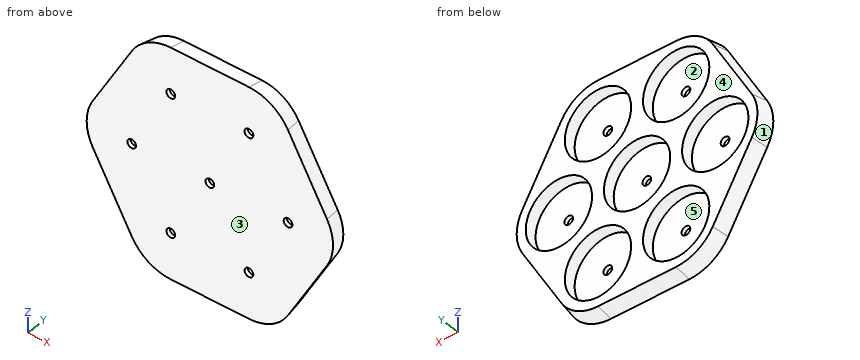
from build123d import *

# Parameters (mm, degrees)
BOSS_EXTRUDE1_DEPTH = 4
BOSS_EXTRUDE1_TAPER = 10
CUT_EXTRUDE1_START  = 4
SKETCH1_3_R         = 1.1
CUT_EXTRUDE1_DEPTH  = 4
CUT_EXTRUDE2_START  = 4
SKETCH1_4_R         = 8.4
SKETCH1_4_R_2       = 1.1
CUT_EXTRUDE2_DEPTH  = 3


with BuildPart() as part:
    # Sketch1 → Boss-Extrude1 (new body)
    with BuildSketch(Plane(origin=(0, 0, 0), x_dir=(1, 0, 0), z_dir=(0, 1, 0))):
        with BuildLine():
            ThreePointArc((-29.7, 28.547302995), (-35.4, 27.019992598), (-39.572689603, 22.847302995))
            Line((-39.572689603, 22.847302995), (-49.472689603, 5.7))
            ThreePointArc((-49.472689603, 5.7), (-51, 0), (-49.472689603, -5.7))
            Line((-49.472689603, -5.7), (-39.572689603, -22.847302995))
            ThreePointArc((-39.572689603, -22.847302995), (-35.4, -27.019992598), (-29.7, -28.547302995))
            Line((-29.7, -28.547302995), (-9.9, -28.547302995))
            ThreePointArc((-9.9, -28.547302995), (-4.2, -27.019992598), (-0.027310397, -22.847302995))
            Line((-0.027310397, -22.847302995), (9.872689603, -5.7))
            ThreePointArc((9.872689603, -5.7), (11.4, 0), (9.872689603, 5.7))
            Line((9.872689603, 5.7), (-0.027310397, 22.847302995))
            ThreePointArc((-0.027310397, 22.847302995), (-4.2, 27.019992598), (-9.9, 28.547302995))
            Line((-9.9, 28.547302995), (-29.7, 28.547302995))
        make_face()
    extrude(amount=BOSS_EXTRUDE1_DEPTH, taper=BOSS_EXTRUDE1_TAPER)

    # Sketch1<3> → Cut-Extrude1 (cut)
    with BuildSketch(Plane(origin=(0, 0, 0), x_dir=(1, 0, 0), z_dir=(0, 1, 0)).offset(CUT_EXTRUDE1_START)):
        with Locations(Location((-9.9, -17.147302995, 0), (0, 0, 270))):
            Circle(SKETCH1_3_R)
        with Locations(Location((0, 0, 0), (0, 0, 270))):
            Circle(SKETCH1_3_R)
        with Locations(Location((-29.7, -17.147302995, 0), (0, 0, 270))):
            Circle(SKETCH1_3_R)
        with Locations(Location((-39.6, 0, 0), (0, 0, 270))):
            Circle(SKETCH1_3_R)
        with Locations(Location((-9.9, 17.147302995, 0), (0, 0, 270))):
            Circle(SKETCH1_3_R)
        with Locations(Location((-29.7, 17.147302995, 0), (0, 0, 270))):
            Circle(SKETCH1_3_R)
        with Locations(Location((-19.8, 0, 0), (0, 0, 270))):
            Circle(SKETCH1_3_R)
    extrude(amount=-CUT_EXTRUDE1_DEPTH, mode=Mode.SUBTRACT)

    # Sketch1<4> → Cut-Extrude2 (cut)
    # profile 1 of 7: a face of its own
    with BuildSketch(Plane(origin=(0, 0, 0), x_dir=(1, 0, 0), z_dir=(0, 1, 0)).offset(CUT_EXTRUDE2_START)):
        with Locations(Location((-19.8, 0, 0), (0, 0, 270))):
            Circle(SKETCH1_4_R)
        with Locations(Location((-19.8, 0, 0), (0, 0, 270))):
            Circle(SKETCH1_4_R_2, mode=Mode.SUBTRACT)
    # profile 2 of 7: a face of its own
    with BuildSketch(Plane(origin=(0, 0, 0), x_dir=(1, 0, 0), z_dir=(0, 1, 0)).offset(CUT_EXTRUDE2_START)):
        with Locations(Location((-9.9, -17.147302995, 0), (0, 0, 270))):
            Circle(SKETCH1_4_R)
        with Locations(Location((-9.9, -17.147302995, 0), (0, 0, 270))):
            Circle(SKETCH1_4_R_2, mode=Mode.SUBTRACT)
    # profile 3 of 7: a face of its own
    with BuildSketch(Plane(origin=(0, 0, 0), x_dir=(1, 0, 0), z_dir=(0, 1, 0)).offset(CUT_EXTRUDE2_START)):
        with Locations(Location((0, 0, 0), (0, 0, 270))):
            Circle(SKETCH1_4_R)
        with Locations(Location((0, 0, 0), (0, 0, 270))):
            Circle(SKETCH1_4_R_2, mode=Mode.SUBTRACT)
    # profile 4 of 7: a face of its own
    with BuildSketch(Plane(origin=(0, 0, 0), x_dir=(1, 0, 0), z_dir=(0, 1, 0)).offset(CUT_EXTRUDE2_START)):
        with Locations(Location((-29.7, -17.147302995, 0), (0, 0, 270))):
            Circle(SKETCH1_4_R)
        with Locations(Location((-29.7, -17.147302995, 0), (0, 0, 270))):
            Circle(SKETCH1_4_R_2, mode=Mode.SUBTRACT)
    # profile 5 of 7: a face of its own
    with BuildSketch(Plane(origin=(0, 0, 0), x_dir=(1, 0, 0), z_dir=(0, 1, 0)).offset(CUT_EXTRUDE2_START)):
        with Locations(Location((-39.6, 0, 0), (0, 0, 270))):
            Circle(SKETCH1_4_R)
        with Locations(Location((-39.6, 0, 0), (0, 0, 270))):
            Circle(SKETCH1_4_R_2, mode=Mode.SUBTRACT)
    # profile 6 of 7: a face of its own
    with BuildSketch(Plane(origin=(0, 0, 0), x_dir=(1, 0, 0), z_dir=(0, 1, 0)).offset(CUT_EXTRUDE2_START)):
        with Locations(Location((-9.9, 17.147302995, 0), (0, 0, 270))):
            Circle(SKETCH1_4_R)
        with Locations(Location((-9.9, 17.147302995, 0), (0, 0, 270))):
            Circle(SKETCH1_4_R_2, mode=Mode.SUBTRACT)
    # profile 7 of 7: a face of its own
    with BuildSketch(Plane(origin=(0, 0, 0), x_dir=(1, 0, 0), z_dir=(0, 1, 0)).offset(CUT_EXTRUDE2_START)):
        with Locations(Location((-29.7, 17.147302995, 0), (0, 0, 270))):
            Circle(SKETCH1_4_R)
        with Locations(Location((-29.7, 17.147302995, 0), (0, 0, 270))):
            Circle(SKETCH1_4_R_2, mode=Mode.SUBTRACT)
    extrude(amount=-CUT_EXTRUDE2_DEPTH, mode=Mode.SUBTRACT)


solid = part.part
Part model, mm, in its own coordinate system. Face numbers are marked on the shaded views. A direction names the side the tool comes from. Coordinates: 2 decimals unless noted, no trailing zeros. Loops run counter-clockwise (first coordinate to the right, second up) from the corner with the lowest first, then second, coordinate; pieces in that order, holes last. Notation, with made-up numbers: M 4,-38 L 23,-38 A10 ccw 23,-21 Z; hole C 44,-16 d10. An arc over 180 degrees is marked long. Use a Markdown table: item, result. Add a question column.
Q1. Cut at B-B (y = 3). Give the number of separate pieces and of enclosed holes in the cut face, and give its area (3 significant figures).
Q2. Which spindle directions (+Z, -Z, +X, -X, +Y, -Y) get a long thin tool onto all of the face, cutting with end or side? Do the marked faces 4 and 5. Say none if no direction does.
Q3. Pin check, flat tips, straight feed: P1, Ø5, axis at x = -17.5, z = -1, coming from the +Y side; P2, Ø2, axis at y = 0.5, z = -21.5, coming from the +X side; P3, Ø1, axis at y = 2, z = -8, coming from the +X side. Stop position of each tip, or through.
Q4. Cut at A-A (z = 0). Write the cut outline in (x, y).
Q5. Mould opens along Z. For the marked faces 1, 2 and 3 say: +Z half, -Z half, draft (parallel to the pull), parting line (faces both ways), or undercut.
Q6. Probe L1, parallel to Z at x = -29, y = 3.8; L2, parallel to X at y = 3.1, z = 0; L3, parallel to Z at x = -24.5, y = 3.8. List the from-to ranges inside material, lowest first.
Worked out:
| question | item | result |
|---|---|---|
| 1 | separate pieces | 1 |
| 1 | enclosed holes | 7 |
| 1 | area | 1,130 mm2 |
| 2 | face 4 | +Z, -Z, +X, -X, +Y |
| 2 | face 5 | +Y |
| 3 | P1 | stops at y = 1 |
| 3 | P2 | stops at x = 1.26 |
| 3 | P3 | stops at x = 8.44 |
| 4 | outline | M -51,0 L -40.7,0 L -40.7,1 L -48,1 L -48,4 L -50.29,4 Z; M -38.5,0 L -20.9,0 L -20.9,1 L -28.2,1 L -28.2,4 L -31.2,4 L -31.2,1 L -38.5,1 Z; M -18.7,0 L -1.1,0 L -1.1,1 L -8.4,1 L -8.4,4 L -11.4,4 L -11.4,1 L -18.7,1 Z; M 1.1,0 L 11.4,0 L 10.69,4 L 8.4,4 L 8.4,1 L 1.1,1 Z |
| 5 | face 1 | parting line |
| 5 | face 2 | undercut |
| 5 | face 3 | draft |
| 6 | L1 | z = -27.88 to -25.52, -8.78 to 8.78, 25.52 to 27.88 |
| 6 | L2 | x = -50.45 to -48, -31.2 to -28.2, -11.4 to -8.4, 8.4 to 10.85 |
| 6 | L3 | z = -27.88 to -23.74, -10.55 to -6.96, 6.96 to 10.55, 23.74 to 27.88 |
